```python
from build123d import *

# Parameters (mm, degrees)
F0_W     = 25.4
F0_H     = 25.4
F1_DEPTH = 2.54
F2_W     = 14.986
F2_H     = 14.986
F3_DEPTH = 76.2
F4_R     = 1.26999


# Not quite as in the source:
# - a fillet or chamfer is up to 0.001 mm smaller than in the source, because OpenCascade refuses the exact size


with BuildPart() as f1:
    # F0 (on Front) → F1 (new body)
    with BuildSketch(Plane.XZ):
        Rectangle(F0_W, F0_H)
    extrude(amount=F1_DEPTH)

    # F2 (on face) → F3 (join)
    with BuildSketch(Plane.XZ.offset(2.54)):
        Rectangle(F2_W, F2_H)
    extrude(amount=F3_DEPTH)

    # F4 (radius 1.27 in the source; OpenCascade refuses exactly that, so slightly less here)
    f4_edges = [f1.edges().sort_by_distance(p)[0] for p in [
        (0, 0, 12.7),
        (-12.7, 0, 0),
        (0, 0, -12.7),
        (12.7, 0, 0),
        (0, -2.54, 12.7),
        (12.7, -2.54, 0),
        (-12.7, -2.54, 0),
        (0, -2.54, -12.7),
        (0, -2.54, 7.493),
        (-7.493, -2.54, 0),
        (0, -2.54, -7.493),
        (7.493, -2.54, 0),
    ]]
    fillet(f4_edges, radius=F4_R)


solid = f1.part
```
Source: CAD feature listing. Evaluate the final solid. Frame: model axes, mm. A direction names the side the tool comes from. Give positions to 0.01 mm unless a question says otherwise; leave off trailing zeros. Loops run counter-clockwise (first coordinate to the right, second up) from the corner with the lowest first, then second, coordinate; pieces in that order, holes last. Notation, with made-up numbers: (37, 14.25) - (61, 14.25) arc R34 cw to (61, 50.25) - close; hole circle Ø8 at (-4, -14). An arc over 180 degrees is marked (long way). Use CSV: the item, a comma, the result in double quotes.
1) Cut plane C-C (y = -16). Output: boundary loops of the cut face in (x, z), and give its area (3 significant figures).
Worked out:
outline,"(-7.49, -7.49) - (7.49, -7.49) - (7.49, 7.49) - (-7.49, 7.49) - close"
area,"225 mm^2"
2) Set-up query: faces 1 (the flat face through (-7.493, -41, 0)), 2 (the flat face through (0, -41, -7.493)), 3 (the flat face through (-10, -2.54, 0)), 4 (the flat face through (7.493, -41, 0)). Return all of +Z, -Z, +X, -X, +Y, -Y with unobstructed straight access to the full face (end or side cutting, diameter ignored); none if empty.
Worked out:
face 1,"+Z, -Z, -X, -Y"
face 2,"-Z, +X, -X, -Y"
face 3,"-Y"
face 4,"+Z, -Z, +X, -Y"
3) Pin query (flat end, axial travel): P1, Ø10, axis at y = -16, z = -1.5, coming from the -X side; P2, Ø6, axis at x = -9, y = -47, coming from the -Z side; P3, Ø12, axis at y = -65.5, z = 3.5, coming from the +X side. Return the tip coordinate at first contact, or that it passes through.
Worked out:
P1,"stops at x = -7.49"
P2,"stops at z = -7.49"
P3,"stops at x = 7.49"
4) Line query: line 1 (X direction, y = -46, z = 5.25); line 2 (Y direction, x = -1.75, z = -10.75). Output: solid intervals per line, ascending.
Worked out:
line 1,"x = -7.49 to 7.49"
line 2,"y = -2.54 to 0"
